Can you work these out from the model? Positions are in its coordinate system, mm. Coordinates: 2 decimals unless noted, no trailing zeros. Loops run counter-clockwise (first coordinate to the right, second up) from the corner with the lowest first, then second, coordinate; pieces in that order, holes last.
```python
from build123d import *

# Parameters (mm, degrees)
F1_DEPTH = 1
F2_R     = 0.9
F2_R_2   = 0.3
F3_DEPTH = 2.001
F4_R     = 2


# Not quite as in the source:
# - a feature names something its author has since deleted; it is built from what else it names


with BuildPart() as f1:
    # F0 (on Front) → F1 (new body, symmetric)
    with BuildSketch(Plane.XZ):
        with BuildLine():
            ThreePointArc((-0.9457076356, 5.3250185657), (-0.1647609851, 4.0136664774), (1, 5))
            ThreePointArc((1, 5), (0.9863335226, 5.1647609851), (0.9457076356, 5.3250185657))
            ThreePointArc((0.9457076356, 5.3250185657), (0, 6), (-0.9457076356, 5.3250185657))
        make_face()
        with BuildLine():
            ThreePointArc((0.9457076356, 5.3250185657), (0.9863335226, 5.1647609851), (1, 5))
            ThreePointArc((1, 5), (-0.1647609851, 4.0136664774), (-0.9457076356, 5.3250185657))
            Line((-0.9457076356, 5.3250185657), (-4.5916600475, -5.2836216754))
            ThreePointArc((-4.5916600475, -5.2836216754), (0, -6.9972097643), (4.5916600475, -5.2836216754))
            Line((4.5916600475, -5.2836216754), (0.9457076356, 5.3250185657))
        make_face()
    extrude(amount=F1_DEPTH, both=True)

    # F2 (on face) → F3 (cut, through all)
    with BuildSketch(Plane.XZ.offset(1)):
        Circle(F2_R)
        with Locations((0, 5)):
            Circle(F2_R_2)
    extrude(amount=-F3_DEPTH, mode=Mode.SUBTRACT)

    # F4
    f4_edges = [f1.edges().sort_by_distance(p)[0] for p in [
        (4.59166, 0, -5.283622),
        (-4.59166, 0, -5.283622),
    ]]
    fillet(f4_edges, radius=F4_R)


solid = f1.part
```
(1) I want a section at C-C on y = -0.35. Write out the boundary of the cut face in (x, z).
Check values:
outline: (-4.09, -3.84) arc R2 ccw to (-3.08, -6.28) arc R7.01 ccw to (3.08, -6.28) arc R2 ccw to (4.09, -3.84) - (0.95, 5.33) arc R1 ccw to (-0.95, 5.33) - close; hole circle Ø1.8 at (0, 0); hole circle Ø0.6 at (0, 5)
(2) I want a section at D-D on z = 5. Write out the boundary of the cut face in (x, y), then the cut area to 3 significant figures.
Check values:
outline: (-1.06, -1) - (-0.3, -1) - (-0.3, 1) - (-1.06, 1) - close; (0.3, -1) - (1.06, -1) - (1.06, 1) - (0.3, 1) - close
area: 3.03 mm2
(3) If I drill on probe 1 along Z at (x, y) = (0, 0.6); probe 2 along Z at (x, y) = (-0.5, 0.65); probe 3 along X at (y, z) = (0.95, -1.5), over which ranges is the centre line in solid material (lowest first)?
Check values:
probe 1: z = -7 to -0.9, 0.9 to 4.7, 5.3 to 6
probe 2: z = -6.98 to -0.75, 0.75 to 5.87
probe 3: x = -3.29 to 3.29
(4) I want a section at A-A on x = 0. Write out the boundary of the cut face in (y, z).
Check values:
outline: (-1, -7) - (1, -7) - (1, -0.9) - (-1, -0.9) - close; (-1, 0.9) - (1, 0.9) - (1, 4.7) - (-1, 4.7) - close; (-1, 5.3) - (1, 5.3) - (1, 6) - (-1, 6) - close
(5) I want a section at B-B on z = 0. Write out the boundary of the cut face in (x, y).
Check values:
outline: (-2.78, -1) - (-0.9, -1) - (-0.9, 1) - (-2.78, 1) - close; (0.9, -1) - (2.78, -1) - (2.78, 1) - (0.9, 1) - close
(6) If we mould it in two halves opening along Z, with no side actions, what happens to faces 1 (the flat face through (0, 1, -2)), 2 (the flat face through (-2.5, 0, 0.8)), 3 (the cylindrical face through (0.86, -0.01, 0.27))? For each: released by +Z, released by -Z, zero draft, split by the parting line, or undercut.
Check values:
face 1: zero draft
face 2: released by +Z
face 3: undercut
